Read the model definition and answer for the solid it produces. Units are mm, in the model's axes. Face numbers are marked on the shaded views. A direction names the side the tool comes from. Round coordinates to 2 decimals unless told otherwise and drop trailing zeros. Write each loop counter-clockwise with the first axis right and the second up, starting at its lowest first coordinate (ties: lowest second). Pieces come first, ordered by that corner, then holes. Notation, with made-up numbers: (-1, -6) -> (30, -6) arc R20 cw to (30, 5) -> close; hole circle Ø8 at (-25.75, 9.25). An arc over 180 degrees is marked (long way). Return JSON: item names as keys, results as strings.
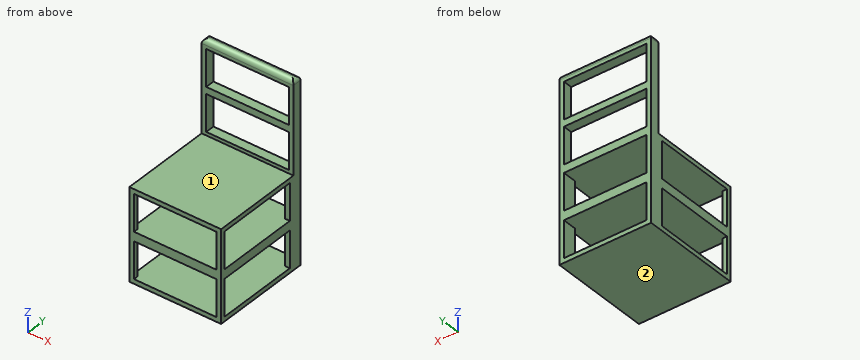
from build123d import *

# Parameters (mm, degrees)
F0_W     = 50
F0_H     = 5
F1_DEPTH = 100
F0_H_2   = 50
F2_DEPTH = 50
F3_W     = 22.5
F3_H     = 20
F4_DEPTH = 100
F5_W     = 22.5
F5_H     = 20
F6_DEPTH = 55
F7_R     = 2.49999
F8_W     = 45
F8_H     = 20
F9_DEPTH = 25


# Not quite as in the source:
# - a fillet or chamfer is up to 0.001 mm smaller than in the source, because OpenCascade refuses the exact size


with BuildPart() as f1:
    # F0 (on Top) → F1 (new body)
    with BuildSketch(Plane.XY):
        with Locations((0, 27.5)):
            Rectangle(F0_W, F0_H)
    extrude(amount=F1_DEPTH)

    # F0 (on Top) → F2 (join)
    with BuildSketch(Plane.XY):
        Rectangle(F0_W, F0_H_2)
    extrude(amount=F2_DEPTH)

    # F3 (on face) → F4 (cut)
    with BuildSketch(Plane.XZ.offset(25)):
        with Locations((-11.25, 37.5)):
            Rectangle(F3_W, F3_H)
        with Locations((11.25, 37.5)):
            Rectangle(F3_W, F3_H)
        with Locations((-11.25, 12.5)):
            Rectangle(F3_W, F3_H)
        with Locations((11.25, 12.5)):
            Rectangle(F3_W, F3_H)
    extrude(amount=-F4_DEPTH, mode=Mode.SUBTRACT)

    # F5 (on face) → F6 (cut)
    with BuildSketch(Plane(origin=(-25, 0, 0), x_dir=(0, -1, 0), z_dir=(-1, 0, 0))):
        with Locations((-11.25, 37.5)):
            Rectangle(F5_W, F5_H)
        with Locations((11.25, 37.5)):
            Rectangle(F5_W, F5_H)
        with Locations((11.25, 12.5)):
            Rectangle(F5_W, F5_H)
        with Locations((-11.25, 12.5)):
            Rectangle(F5_W, F5_H)
    extrude(amount=-F6_DEPTH, mode=Mode.SUBTRACT)

    # F7 (radius 2.5 in the source; OpenCascade refuses exactly that, so slightly less here)
    f7_edges = [f1.edges().sort_by_distance(p)[0] for p in [
        (0, 25, 100),
        (25, 27.5, 100),
        (0, 30, 100),
        (-25, 27.5, 100),
    ]]
    fillet(f7_edges, radius=F7_R)

    # F8 (on face) → F9 (cut)
    with BuildSketch(Plane.XZ.offset(-25)):
        with Locations((0, 85.625)):
            Rectangle(F8_W, F8_H)
        with Locations((0, 61.875)):
            Rectangle(F8_W, F8_H)
    extrude(amount=-F9_DEPTH, mode=Mode.SUBTRACT)


solid = f1.part
Item 1: Section C-C (y = 1) is taken. Give the vertices of the cut face in (x, z).
Worked answers:
{"outline": "(-25, 0) -> (25, 0) -> (25, 2.5) -> (-25, 2.5) -> close; (-25, 22.5) -> (25, 22.5) -> (25, 27.5) -> (-25, 27.5) -> close; (-25, 47.5) -> (25, 47.5) -> (25, 50) -> (-25, 50) -> close"}
Item 2: Straight lines are drawn through the part: L1, parallel to Z at x = 12.5, y = -21; L2, parallel to X at y = 23, z = 40; L3, parallel to Y at x = -10.5, z = 51.5. For each, find the intervals that lie inside material, in ascending order. Write a range as [from, to].
Worked answers:
{"L1": "z = [0, 2.5], [22.5, 27.5], [47.5, 50]", "L2": "x = [-25, -22.5], [22.5, 25]", "L3": "y = [25, 30]"}
Item 3: A flat-ended cylindrical pin translates along its axis: pin 1 (15 mm diameter, centred on x = -6, y = -1, fed in from +Z). Find the tip coordinate at first contact, or state that the pin passes through.
Worked answers:
{"pin 1": "stops at z = 50"}
Item 4: Section A-A (z = 85) is taken. Give the vertices of the cut face in (x, y).
Worked answers:
{"outline": "(-25, 25) -> (-22.5, 25) -> (-22.5, 30) -> (-25, 30) -> close; (22.5, 25) -> (25, 25) -> (25, 30) -> (22.5, 30) -> close"}
Item 5: Section B-B (x = -8) is taken. State how many separate pieces and enclosed holes the cut face has, then the cut area to 3 significant figures.
Worked answers:
{"separate pieces": "5", "enclosed holes": "0", "area": "597 mm2"}
Item 6: A tool of negligible diameter and unlimited length cuts with its end or side. For the marked faces 1 and 2, from which of +Z, -Z, +X, -X, +Y, -Y can it reach the whole face along a straight path? Write none if from no direction.
Worked answers:
{"face 1": "+Z, +X, -X, -Y", "face 2": "-Z, +X, -X, +Y, -Y"}
